```python
from build123d import *

# Parameters (mm, degrees)
CROQUIS1_W                         = 431.038
CROQUIS1_H                         = 381
BRIDA_BASE1_DEPTH                  = 1.524
CROQUIS6_W                         = 3.048
CROQUIS6_H                         = 3.048
CORTAR_EXTRUIR1_DEPTH              = 288.647374292
BRIDA_DE_ARISTA1_STRIP_W           = 9.144
BRIDA_DE_ARISTA1_STRIP_H           = 1.524
BRIDA_DE_ARISTA1_STRIP_CUT_DEPTH   = 427.99
BRIDA_DE_ARISTA1_STRIP_2_W         = 9.144
BRIDA_DE_ARISTA1_STRIP_2_H         = 1.524
BRIDA_DE_ARISTA1_STRIP_CUT_2_DEPTH = 374.904
BRIDA_DE_ARISTA1_STRIP_3_W         = 9.144
BRIDA_DE_ARISTA1_STRIP_3_H         = 1.524
BRIDA_DE_ARISTA1_STRIP_CUT_3_DEPTH = 427.99
BRIDA_DE_ARISTA1_DEPTH             = 427.99
BRIDA_DE_ARISTA1_BEND_DEPTH        = 374.904
BRIDA_DE_ARISTA1_BEND_2_DEPTH      = 427.99
CROQUIS16_R                        = 3.9624
CROQUIS16_R_2                      = 2.8956
CROQUIS16_R_3                      = 11.176
CROQUIS16_R_4                      = 2.413
CROQUIS16_W                        = 186.944
CROQUIS16_H                        = 138.938
CORTAR_EXTRUIR2_DEPTH              = 289.088100006


# Sheet-metal steps are written as plain solids
with BuildPart() as part:
    # Croquis1 → Brida base1 (new body)
    with BuildSketch(Plane.XY):
        Rectangle(CROQUIS1_W, CROQUIS1_H)
    extrude(amount=-BRIDA_BASE1_DEPTH)

    # Croquis6 → Cortar-Extruir1 (cut, through all)
    with BuildSketch(Plane.XY):
        with Locations((-213.995, 188.976)):
            Rectangle(CROQUIS6_W, CROQUIS6_H)
        with Locations((-213.995, -188.976)):
            Rectangle(CROQUIS6_W, CROQUIS6_H)
    extrude(amount=-CORTAR_EXTRUIR1_DEPTH, mode=Mode.SUBTRACT)

    # Brida de arista1 strip (across the edge) → Brida de arista1 strip cut (cut)
    with BuildSketch(Plane(origin=(-212.471, 190.5, -1.524), x_dir=(0, -1, 0), z_dir=(1, 0, 0))):
        with Locations((-1.524, -0.762)):
            Rectangle(BRIDA_DE_ARISTA1_STRIP_W, BRIDA_DE_ARISTA1_STRIP_H)
    extrude(amount=BRIDA_DE_ARISTA1_STRIP_CUT_DEPTH, mode=Mode.SUBTRACT)

    # Brida de arista1 strip 2 (across the edge) → Brida de arista1 strip cut 2 (cut)
    with BuildSketch(Plane(origin=(-215.519, -187.452, -1.524), x_dir=(1, 0, 0), z_dir=(0, 1, 0))):
        with Locations((-1.524, -0.762)):
            Rectangle(BRIDA_DE_ARISTA1_STRIP_2_W, BRIDA_DE_ARISTA1_STRIP_2_H)
    extrude(amount=BRIDA_DE_ARISTA1_STRIP_CUT_2_DEPTH, mode=Mode.SUBTRACT)

    # Brida de arista1 strip 3 (across the edge) → Brida de arista1 strip cut 3 (cut)
    with BuildSketch(Plane(origin=(215.519, -190.5, -1.524), x_dir=(0, 1, 0), z_dir=(-1, 0, 0))):
        with Locations((-1.524, -0.762)):
            Rectangle(BRIDA_DE_ARISTA1_STRIP_3_W, BRIDA_DE_ARISTA1_STRIP_3_H)
    extrude(amount=BRIDA_DE_ARISTA1_STRIP_CUT_3_DEPTH, mode=Mode.SUBTRACT)

    # Brida de arista1 section (across the edge) → Brida de arista1 (add)
    with BuildSketch(Plane(origin=(-212.471, 190.5, -1.524), x_dir=(0, -1, 0), z_dir=(1, 0, 0))):
        with BuildLine():
            Line((0, 1.524), (0, 14.478))
            Line((0, 14.478), (1.524, 14.478))
            Line((1.524, 14.478), (1.524, 1.524))
            ThreePointArc((1.524, 1.524), (1.970369265, 0.446369265), (3.048, 0))
            Line((3.048, 0), (3.048, -1.524))
            ThreePointArc((3.048, -1.524), (0.892738531, -0.631261469), (0, 1.524))
        make_face()
    extrude(amount=BRIDA_DE_ARISTA1_DEPTH)

    # Brida de arista1 section 2 (across the edge) → Brida de arista1 bend (add)
    with BuildSketch(Plane(origin=(-215.519, -187.452, -1.524), x_dir=(1, 0, 0), z_dir=(0, 1, 0))):
        with BuildLine():
            Line((0, 1.524), (0, 14.478))
            Line((0, 14.478), (1.524, 14.478))
            Line((1.524, 14.478), (1.524, 1.524))
            ThreePointArc((1.524, 1.524), (1.970369265, 0.446369265), (3.048, 0))
            Line((3.048, 0), (3.048, -1.524))
            ThreePointArc((3.048, -1.524), (0.892738531, -0.631261469), (0, 1.524))
        make_face()
    extrude(amount=BRIDA_DE_ARISTA1_BEND_DEPTH)

    # Brida de arista1 section 3 (across the edge) → Brida de arista1 bend 2 (add)
    with BuildSketch(Plane(origin=(215.519, -190.5, -1.524), x_dir=(0, 1, 0), z_dir=(-1, 0, 0))):
        with BuildLine():
            Line((0, 1.524), (0, 14.478))
            Line((0, 14.478), (1.524, 14.478))
            Line((1.524, 14.478), (1.524, 1.524))
            ThreePointArc((1.524, 1.524), (1.970369265, 0.446369265), (3.048, 0))
            Line((3.048, 0), (3.048, -1.524))
            ThreePointArc((3.048, -1.524), (0.892738531, -0.631261469), (0, 1.524))
        make_face()
    extrude(amount=BRIDA_DE_ARISTA1_BEND_2_DEPTH)

    # Croquis16 → Cortar-Extruir2 (cut, through all)
    with BuildSketch(Plane.XY):
        with Locations((-202.819, 0)):
            Circle(CROQUIS16_R)
        with Locations((-167.767, 60.452)):
            Circle(CROQUIS16_R_2)
        with Locations((-167.767, -60.452)):
            Circle(CROQUIS16_R_2)
        with Locations((-50.165, -127)):
            Circle(CROQUIS16_R_3)
        with Locations((51.435, -127)):
            Circle(CROQUIS16_R_3)
        with Locations((207.645, 152.4)):
            Circle(CROQUIS16_R_4)
        with Locations((207.645, 0)):
            Circle(CROQUIS16_R_4)
        with Locations((207.645, -152.4)):
            Circle(CROQUIS16_R_4)
        with Locations((-0.127, 0)):
            Rectangle(CROQUIS16_W, CROQUIS16_H)
    extrude(amount=-CORTAR_EXTRUIR2_DEPTH, mode=Mode.SUBTRACT)


solid = part.part
```
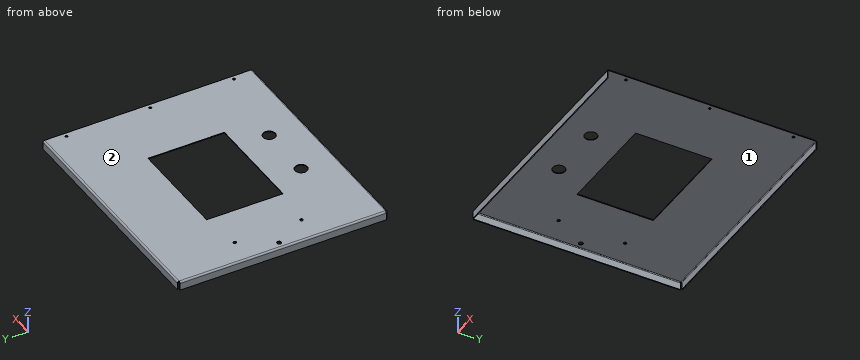
The listing builds one solid part. Answer for the finished solid, in the listing's coordinates (mm). Face numbers are marked on the shaded views. A direction names the side the tool comes from. Give positions to 0.01 mm unless a question says otherwise; leave off trailing zeros. Order: outer loops, then holes, each group sorted by start corner. A loop starts at its lowest first (then second) coordinate and runs counter-clockwise, first axis right, second up.
1) Find section A-A on y = -127. Write down the section's boundary in (x, z) (3 decimals).
Reported:
outline: (-215.519, -16.002) - (-213.995, -16.002) - (-213.995, -3.048) arc R1.524 cw to (-212.471, -1.524) - (-61.341, -1.524) - (-61.341, 0) - (-212.471, 0) arc R3.048 ccw to (-215.519, -3.048) - close; (-38.989, -1.524) - (40.259, -1.524) - (40.259, 0) - (-38.989, 0) - close; (62.611, -1.524) - (215.519, -1.524) - (215.519, 0) - (62.611, 0) - close
2) Find section B-B on x = 79. Write down the section's boundary in (y, z).
Reported:
outline: (-190.5, -16) - (-188.98, -16) - (-188.98, -3.05) arc R1.52 cw to (-187.45, -1.52) - (-69.47, -1.52) - (-69.47, 0) - (-187.45, 0) arc R3.05 ccw to (-190.5, -3.05) - close; (69.47, -1.52) - (187.45, -1.52) arc R1.52 cw to (188.98, -3.05) - (188.98, -16) - (190.5, -16) - (190.5, -3.05) arc R3.05 ccw to (187.45, 0) - (69.47, 0) - close
3) For the marked faces 1 and 2, determine the directions among +Z, -Z, +X, -X, +Y, -Y from which every point of the face is accessible in a straight line to the end or side of a thin tool.
Reported:
face 1: -Z, +X
face 2: +Z, +X, -X, +Y, -Y
4) Find section C-C on y = -40. Write down the section's boundary in (x, z) (3 decimals).
Reported:
outline: (-215.519, -16.002) - (-213.995, -16.002) - (-213.995, -3.048) arc R1.524 cw to (-212.471, -1.524) - (-93.599, -1.524) - (-93.599, 0) - (-212.471, 0) arc R3.048 ccw to (-215.519, -3.048) - close; (93.345, -1.524) - (215.519, -1.524) - (215.519, 0) - (93.345, 0) - close
5) Given P1, Ø3, axis at x = 207.645, y = 152.4, coming from the -Z side; P2, Ø5.5, axis at x = 207.645, y = -152.4, coming from the -Z side; P3, Ø2.5, axis at x = -214, z = -5, coming from the +Y side; P4, Ø6.5, axis at y = 70.5, z = -11, coming from the +X side (3 decimals), each flat-ended and moving along its own axis, determine where each tip first touches the part or whether it passes through.
Reported:
P1: passes through
P2: stops at z = -1.52
P3: stops at y = 187.45
P4: stops at x = -213.995
6) Consider line 1 along Y through (x, z) = (96.5, -9.75); line 2 along X through (y, z) = (-152.4, -0.4); line 3 along Z through (x, y) = (-56.5, -76). Determine where each line is inside the solid, lowest interval first.
Reported:
line 1: y = -190.5 to -188.98, 188.98 to 190.5
line 2: x = -213.98 to 205.23, 210.06 to 215.52
line 3: z = -1.52 to 0
7) Find section D-D on z = -13.25. Write down the section's boundary in (x, y) (3 decimals), then the cut area to 3 significant figures.
Reported:
outline: (-215.519, -187.452) - (-213.995, -187.452) - (-213.995, 187.452) - (-215.519, 187.452) - close; (-212.471, -190.5) - (215.519, -190.5) - (215.519, -188.976) - (-212.471, -188.976) - close; (-212.471, 188.976) - (215.519, 188.976) - (215.519, 190.5) - (-212.471, 190.5) - close
area: 1,880 mm2
